Check sheet for the modelled part. Datum: model origin and axes. Units: mm. A direction names the side the tool comes from. Give positions to 0.01 mm unless a question says otherwise; leave off trailing zeros. Write each loop counter-clockwise with the first axis right and the second up, starting at its lowest first coordinate (ties: lowest second). Pieces come first, ordered by that corner, then holes.
from build123d import *

# Parameters (mm, degrees)
BOSS_EXTRUDE1_DEPTH = 40
CUT_EXTRUDE1_DEPTH  = 22.857142857


with BuildPart() as part:
    # Sketch2 → Boss-Extrude1 (new body)
    with BuildSketch(Plane(origin=(0, 0, 0), x_dir=(1, 0, 0), z_dir=(0, 1, 0))):
        with BuildLine():
            Line((0, 2.775), (3.1979918, 3))
            Line((3.1979918, 3), (4.769352085, 3))
            ThreePointArc((4.769352085, 3), (4.275, 0), (4.769352085, -3))
            Line((4.769352085, -3), (3.1979918, -3))
            Line((3.1979918, -3), (0, -2.775))
            ThreePointArc((0, -2.775), (-2.775, 0), (0, 2.775))
        make_face()
        with BuildLine():
            Line((0, 1.65), (2.935008537, 1.856497378))
            ThreePointArc((2.935008537, 1.856497378), (2.775, 0), (2.935008537, -1.856497378))
            Line((2.935008537, -1.856497378), (0, -1.65))
            ThreePointArc((0, -1.65), (-1.65, 0), (0, 1.65))
        make_face(mode=Mode.SUBTRACT)
    extrude(amount=BOSS_EXTRUDE1_DEPTH)

    # Sketch3 → Cut-Extrude1 (cut)
    with BuildSketch(Plane(origin=(0, 40, 0), x_dir=(1, 0, 0), z_dir=(0, 1, 0))):
        with BuildLine():
            Line((3.675, 1.55), (4.404370954, 1.55))
            ThreePointArc((4.404370954, 1.55), (4.275, 0), (4.404370954, -1.55))
            Line((4.404370954, -1.55), (3.675, -1.55))
            Line((3.675, -1.55), (3.675, 1.55))
        make_face()
    extrude(amount=-CUT_EXTRUDE1_DEPTH, mode=Mode.SUBTRACT)


solid = part.part
1) Sectioned sample at C-C on x = 1.75. Record the boundary of the cut face in (y, z), then the cut area to 3 significant figures.
2) Draft check along Z on faces 4 (the flat face through (4, 20, 3)), 5 (the flat face through (1.488, 19.72, 1.755)), 6 (the flat face through (1.577, 19.72, -2.886)), 7 (the flat face through (1, 40, 2)). Enter one of: +Z half, -Z half, draft (parallel to the pull), parting line (faces both ways), or undercut.
3) Access from +Z, -Z, +X, -X, +Y, -Y to the whole of each face (thin tool, end or side, straight path). Record for faces 1 (the flat face through (3.675, 29, 0)), 2 (the flat face through (1.447, 19.72, -1.752)), 3 (the flat face through (1, 0, 2)).
4) Gauge pin test, flat ends, axial feed: pin 1 (2 mm diameter, centred on y = 9.5, z = -1, fed in from +X); pin 2 (1.6 mm diameter, centred on y = 26.5, z = 0.5, fed in from +X) (3 decimals); pin 3 (2 mm diameter, centred on y = 25, z = 1.5, fed in from -X). Record the tip position at first contact, or that the pin passes through.
5) Scan lines: L1, parallel to X at y = 5.5, z = 0.75; L2, parallel to X at y = 3, z = 1; L3, parallel to Z at x = -1, y = 27. Record each from-to range of solid material in increasing order.
6) Sectioned sample at A-A on z = 0. Record the boundary of the cut face in (x, y) (3 decimals).
Answers below:
1. outline: (0, -2.9) - (40, -2.9) - (40, -1.77) - (0, -1.77) - close; (0, 1.77) - (40, 1.77) - (40, 2.9) - (0, 2.9) - close
1. area: 90.0 mm2
2. face 4: +Z half
2. face 5: undercut
2. face 6: -Z half
2. face 7: draft
3. face 1: +X, +Y
3. face 2: +Y, -Y
3. face 3: +Z, -Z, +X, -X, -Y
4. pin 1: stops at x = 4.49
4. pin 2: stops at x = 3.675
4. pin 3: stops at x = -2.73
5. L1: x = -2.67 to -1.47, 2.8 to 4.31
5. L2: x = -2.59 to -1.31, 2.82 to 4.33
5. L3: z = -2.59 to -1.31, 1.31 to 2.59
6. outline: (-2.775, 0) - (-1.65, 0) - (-1.65, 40) - (-2.775, 40) - close; (2.775, 0) - (4.275, 0) - (4.275, 17.143) - (3.675, 17.143) - (3.675, 40) - (2.775, 40) - close
